from build123d import *

# Parameters (mm, degrees)
F1_DEPTH     = 3
F2_DEPTH     = 8
F3_R         = 8
F4_T4_DEPTH  = 113.9006842239
F4_T9_ANGLE  = 95
F4_T14_ANGLE = 85
F4_T19_DEPTH = 49.1871720396
F4_T24_ANGLE = 95
F4_T29_DEPTH = 20.662188907
F4_T34_ANGLE = 31.4669762933
F4_T39_ANGLE = 62.9339525865
F4_T44_ANGLE = 31.4669762933
F4_T49_DEPTH = 22.2455379196
F4_T54_ANGLE = 85
F4_T59_DEPTH = 49.1871720396
F5_SIZE      = 1
F6_T1_DEPTH  = 123.9388825993
F6_T3_DEPTH  = 59.2253704151
F6_T5_DEPTH  = 42.8508484491
F6_T7_DEPTH  = 59.2253704151
F6_T9_DEPTH  = 43.5593108265
F6_T12_ANGLE = 96.9904356043
F6_T14_ANGLE = 95
F6_T16_ANGLE = 85
F6_T18_ANGLE = 95
F6_T20_ANGLE = 85


# Not quite as in the source:
# - a fillet or chamfer that OpenCascade refuses, or shapes differently, is made with other operations: its cross-section is extruded or revolved along the edge and cut away or added


with BuildPart() as f1:
    # F0 (on Right) → F1 (new body)
    with BuildSketch(Plane.YZ):
        with BuildLine():
            Line((-76.6886542646, 55.3186824411), (-76.6886542646, -19.9678053747))
            Line((-76.6886542646, -19.9678053747), (-38.1131050777, -16.5928821315))
            ThreePointArc((-38.1131050777, -16.5928821315), (-7.4822201157, -3.8748285682), (24.8917797013, -11.0806689666))
            Line((24.8917797013, -11.0806689666), (62.7786034683, -7.76600139))
            Line((62.7786034683, -7.76600139), (62.7786034683, 67.5204864257))
            Line((62.7786034683, 67.5204864257), (-76.6886542646, 55.3186824411))
        make_face()
        with BuildLine():
            Line((-40.0864817191, -11.7464310288), (-71.6886542646, -14.5112628693))
            Line((-71.6886542646, -14.5112628693), (-71.6886542646, 50.737026571))
            Line((-71.6886542646, 50.737026571), (57.7786034683, 62.0639439204))
            Line((57.7786034683, 62.0639439204), (57.7786034683, -3.1843455199))
            Line((57.7786034683, -3.1843455199), (25.9935989152, -5.9651730884))
            ThreePointArc((25.9935989152, -5.9651730884), (-7.9179988294, 1.1061449223), (-40.0864817191, -11.7464310288))
        make_face(mode=Mode.SUBTRACT)
        with BuildLine():
            Line((-71.6886542646, 50.737026571), (-71.6886542646, -14.5112628693))
            Line((-71.6886542646, -14.5112628693), (-40.0864817191, -11.7464310288))
            ThreePointArc((-40.0864817191, -11.7464310288), (-7.9179988294, 1.1061449223), (25.9935989152, -5.9651730884))
            Line((25.9935989152, -5.9651730884), (57.7786034683, -3.1843455199))
            Line((57.7786034683, -3.1843455199), (57.7786034683, 62.0639439204))
            Line((57.7786034683, 62.0639439204), (-71.6886542646, 50.737026571))
        make_face()
    extrude(amount=-F1_DEPTH)

    # F0 (on Right) → F2 (join)
    with BuildSketch(Plane.YZ):
        with BuildLine():
            Line((-71.6886542646, 50.737026571), (-71.6886542646, -14.5112628693))
            Line((-71.6886542646, -14.5112628693), (-40.0864817191, -11.7464310288))
            ThreePointArc((-40.0864817191, -11.7464310288), (-7.9179988294, 1.1061449223), (25.9935989152, -5.9651730884))
            Line((25.9935989152, -5.9651730884), (57.7786034683, -3.1843455199))
            Line((57.7786034683, -3.1843455199), (57.7786034683, 62.0639439204))
            Line((57.7786034683, 62.0639439204), (-71.6886542646, 50.737026571))
        make_face()
    extrude(amount=-F2_DEPTH)

    # F3
    f3_edges = [f1.edges().sort_by_distance(p)[0] for p in [
        (-5.5, 57.778603, 62.063944),
        (-5.5, -71.688654, 50.737027),
        (-5.5, -71.688654, -14.511263),
        (-5.5, -40.086482, -11.746431),
        (-5.5, 25.993599, -5.965173),
        (-5.5, 57.778603, -3.184346),
        (-1.5, -76.688654, 55.318682),
        (-1.5, -76.688654, -19.967805),
        (-1.5, 62.778603, -7.766001),
        (-1.5, 62.778603, 67.520486),
    ]]
    fillet(f3_edges, radius=F3_R)

    # F4: chamfer of 1 x 6 on 1 edges, made by hand


with BuildPart() as f4_tool2:
    # F4_s3 → F4_t4 (new body)
    with BuildSketch(Plane(origin=(0, 54.0311094993, 4.7271095589), x_dir=(1, 0, 0), z_dir=(0, -0.9961946981, -0.0871557427))):
        Polygon((-2, 56.792034776), (-8, 55.792034776), (-8, 56.792034776), align=None)
    extrude(amount=F4_T4_DEPTH)

    split(bisect_by=Plane.YZ.offset(-3), keep=Keep.BOTTOM)


with BuildPart() as f1_1:
    add(f1.part)

    # F4_t1: cut F4_tool2
    add(f4_tool2.part, mode=Mode.SUBTRACT)


with BuildPart() as f4_tool7:
    # F4_s8 → F4_t9 (revolve)
    with BuildSketch(Plane.XY.offset(53.3334759118)):
        Polygon((-2, 57.7786034683), (-8, 56.7786034683), (-8, 57.7786034683), align=None)
    revolve(axis=Axis((-8, 49.7786034683, 53.3334759118), (1, 0, 0)), revolution_arc=F4_T9_ANGLE)

    split(bisect_by=Plane.YZ.offset(-3), keep=Keep.BOTTOM)


with BuildPart() as f1_2:
    add(f1_1.part)

    # F4_t6: cut F4_tool7
    add(f4_tool7.part, mode=Mode.SUBTRACT)


with BuildPart() as f4_tool12:
    # F4_s13 → F4_t14 (revolve)
    with BuildSketch(Plane.XY.offset(43.4063771788)):
        Polygon((-2, -71.6886542646), (-8, -70.6886542646), (-8, -71.6886542646), align=None)
    revolve(axis=Axis((-8, -63.6886542646, 43.4063771788), (-1, 0, 0)), revolution_arc=F4_T14_ANGLE)

    split(bisect_by=Plane.YZ.offset(-3), keep=Keep.BOTTOM)


with BuildPart() as f1_3:
    add(f1_2.part)

    # F4_t11: cut F4_tool12
    add(f4_tool12.part, mode=Mode.SUBTRACT)


with BuildPart() as f4_tool17:
    # F4_s18 → F4_t19 (new body)
    with BuildSketch(Plane.XY.offset(43.4063771788)):
        Polygon((-2, -71.6886542646), (-8, -70.6886542646), (-8, -71.6886542646), align=None)
    extrude(amount=-F4_T19_DEPTH)

    split(bisect_by=Plane.YZ.offset(-3), keep=Keep.BOTTOM)


with BuildPart() as f1_4:
    add(f1_3.part)

    # F4_t16: cut F4_tool17
    add(f4_tool17.part, mode=Mode.SUBTRACT)


with BuildPart() as f4_tool22:
    # F4_s23 → F4_t24 (revolve)
    with BuildSketch(Plane.XY.offset(-5.7807948608)):
        Polygon((-2, -71.6886542646), (-8, -70.6886542646), (-8, -71.6886542646), align=None)
    revolve(axis=Axis((-8, -63.6886542646, -5.7807948608), (1, 0, 0)), revolution_arc=F4_T24_ANGLE)

    split(bisect_by=Plane.YZ.offset(-3), keep=Keep.BOTTOM)


with BuildPart() as f1_5:
    add(f1_4.part)

    # F4_t21: cut F4_tool22
    add(f4_tool22.part, mode=Mode.SUBTRACT)


with BuildPart() as f4_tool27:
    # F4_s28 → F4_t29 (new body)
    with BuildSketch(Plane(origin=(0, -63.7067796281, -5.5736210072), x_dir=(1, 0, 0), z_dir=(0, 0.9961946981, 0.0871557427))):
        Polygon((-2, 8.207965224), (-8, 7.207965224), (-8, 8.207965224), align=None)
    extrude(amount=F4_T29_DEPTH)

    split(bisect_by=Plane.YZ.offset(-3), keep=Keep.BOTTOM)


with BuildPart() as f1_6:
    add(f1_5.part)

    # F4_t26: cut F4_tool27
    add(f4_tool27.part, mode=Mode.SUBTRACT)


with BuildPart() as f4_tool32:
    # F4_s33 → F4_t34 (revolve)
    with BuildSketch(Plane(origin=(0, -43.123216588, -3.7727925862), x_dir=(1, 0, 0), z_dir=(0, -0.9961946981, -0.0871557427))):
        Polygon((-2, -8.207965224), (-8, -7.207965224), (-8, -8.207965224), align=None)
    revolve(axis=Axis((-8, -43.1050912244, -3.9799664398), (1, 0, 0)), revolution_arc=F4_T34_ANGLE)

    split(bisect_by=Plane.YZ.offset(-3), keep=Keep.BOTTOM)


with BuildPart() as f1_7:
    add(f1_6.part)

    # F4_t31: cut F4_tool32
    add(f4_tool32.part, mode=Mode.SUBTRACT)


with BuildPart() as f4_tool37:
    # F4_s38 → F4_t39 (revolve)
    with BuildSketch(Plane(origin=(0, -29.7800133865, -22.0094994379), x_dir=(1, 0, 0), z_dir=(0, -0.8041995665, -0.5943593671))):
        Polygon((-2, 14.4192274514), (-8, 15.4192274514), (-8, 14.4192274514), align=None)
    revolve(axis=Axis((-8, -2.6886542646, -58.6655369632), (-1, 0, 0)), revolution_arc=F4_T39_ANGLE)

    split(bisect_by=Plane.YZ.offset(-3), keep=Keep.BOTTOM)


with BuildPart() as f1_8:
    add(f1_7.part)

    # F4_t36: cut F4_tool37
    add(f4_tool37.part, mode=Mode.SUBTRACT)


with BuildPart() as f4_tool42:
    # F4_s43 → F4_t44 (revolve)
    with BuildSketch(Plane(origin=(0, 21.2512251902, -10.5801809941), x_dir=(1, 0, 0), z_dir=(0, -0.895191389, 0.4456819235))):
        Polygon((-2, 6.2848318723), (-8, 7.2848318723), (-8, 6.2848318723), align=None)
    revolve(axis=Axis((-8, 27.6177165365, 2.207477492), (1, 0, 0)), revolution_arc=F4_T44_ANGLE)

    split(bisect_by=Plane.YZ.offset(-3), keep=Keep.BOTTOM)


with BuildPart() as f1_9:
    add(f1_8.part)

    # F4_t41: cut F4_tool42
    add(f4_tool42.part, mode=Mode.SUBTRACT)


with BuildPart() as f4_tool47:
    # F4_s48 → F4_t49 (new body)
    with BuildSketch(Plane(origin=(0, 27.599591173, 2.4146513456), x_dir=(1, 0, 0), z_dir=(0, 0.9961946981, 0.0871557427))):
        Polygon((-2, 8.207965224), (-8, 7.207965224), (-8, 8.207965224), align=None)
    extrude(amount=F4_T49_DEPTH)

    split(bisect_by=Plane.YZ.offset(-3), keep=Keep.BOTTOM)


with BuildPart() as f1_10:
    add(f1_9.part)

    # F4_t46: cut F4_tool47
    add(f4_tool47.part, mode=Mode.SUBTRACT)


with BuildPart() as f4_tool52:
    # F4_s53 → F4_t54 (revolve)
    with BuildSketch(Plane(origin=(0, 49.7604781047, 4.3534777258), x_dir=(1, 0, 0), z_dir=(0, -0.9961946981, -0.0871557427))):
        Polygon((-2, -8.207965224), (-8, -7.207965224), (-8, -8.207965224), align=None)
    revolve(axis=Axis((-8, 49.7786034683, 4.1463038722), (1, 0, 0)), revolution_arc=F4_T54_ANGLE)

    split(bisect_by=Plane.YZ.offset(-3), keep=Keep.BOTTOM)


with BuildPart() as f1_11:
    add(f1_10.part)

    # F4_t51: cut F4_tool52
    add(f4_tool52.part, mode=Mode.SUBTRACT)


with BuildPart() as f4_tool57:
    # F4_s58 → F4_t59 (new body)
    with BuildSketch(Plane.XY.offset(4.1463038722)):
        Polygon((-2, 57.7786034683), (-8, 56.7786034683), (-8, 57.7786034683), align=None)
    extrude(amount=F4_T59_DEPTH)

    split(bisect_by=Plane.YZ.offset(-3), keep=Keep.BOTTOM)


with BuildPart() as f1_12:
    add(f1_11.part)

    # F4_t56: cut F4_tool57
    add(f4_tool57.part, mode=Mode.SUBTRACT)

    # F5
    f5_edges = [f1_12.edges().sort_by_distance(p)[0] for p in [
        (-8, -7.565116, 55.343289),
        (-8, -68.849596, 48.135509),
        (-8, 54.507735, 58.494417),
        (-8, 54.939545, -0.582828),
        (-8, 39.30825, -3.796472),
        (-8, 26.31403, -4.670051),
        (-8, -8.005155, 2.10234),
        (-8, -40.626941, -10.526627),
        (-8, -52.786783, -11.853744),
        (-8, -68.417786, -10.941736),
        (-8, -70.688654, 18.812791),
        (-8, 56.778603, 28.73989),
    ]]
    chamfer(f5_edges, length=F5_SIZE)

    # F6: chamfer of 5 on 2 edges, made by hand

    # F6_s2 → F6_t1 (cut)
    with BuildSketch(Plane(origin=(0, 59.4668882131, 5.2026785738), x_dir=(1, 0, 0), z_dir=(0, -0.9961946981, -0.0871557427))):
        Polygon((-5, 61.792034776), (0, 56.792034776), (0, 61.792034776), align=None)
    extrude(amount=F6_T1_DEPTH, mode=Mode.SUBTRACT)

    # F6_s4 → F6_t3 (cut)
    with BuildSketch(Plane.XY.offset(-11.2373373661)):
        Polygon((-5, -76.6886542646), (0, -71.6886542646), (0, -76.6886542646), align=None)
    extrude(amount=F6_T3_DEPTH, mode=Mode.SUBTRACT)

    # F6_s6 → F6_t5 (cut)
    with BuildSketch(Plane(origin=(0, -69.1425583419, -6.0491900221), x_dir=(1, 0, 0), z_dir=(0, 0.9961946981, 0.0871557427))):
        Polygon((-5, 13.207965224), (0, 8.207965224), (0, 13.207965224), align=None)
    extrude(amount=F6_T5_DEPTH, mode=Mode.SUBTRACT)

    # F6_s8 → F6_t7 (cut)
    with BuildSketch(Plane.XY.offset(-0.4353519979)):
        Polygon((-5, 62.7786034683), (0, 57.7786034683), (0, 62.7786034683), align=None)
    extrude(amount=F6_T7_DEPTH, mode=Mode.SUBTRACT)

    # F6_s10 → F6_t9 (cut)
    with BuildSketch(Plane(origin=(0, 10.9311448931, 0.9563512575), x_dir=(1, 0, 0), z_dir=(0, 0.9961946981, 0.0871557427))):
        Polygon((-5, 13.207965224), (0, 8.207965224), (0, 13.207965224), align=None)
    extrude(amount=F6_T9_DEPTH, mode=Mode.SUBTRACT)

    # F6_s11 → F6_t12 (revolve, cut)
    with BuildSketch(Plane(origin=(0, -29.0039957446, -39.1898093404), x_dir=(1, 0, 0), z_dir=(0, -0.5948898787, -0.8038072109))):
        Polygon((-5, 22.2616255192), (0, 27.2616255192), (0, 22.2616255192), align=None)
    revolve(axis=Axis((0, -2.6886542646, -58.6655369632), (-1, 0, 0)), revolution_arc=F6_T12_ANGLE, mode=Mode.SUBTRACT)

    # F6_s13 → F6_t14 (revolve, cut)
    with BuildSketch(Plane(origin=(0, 59.4668882131, 5.2026785738), x_dir=(1, 0, 0), z_dir=(0, -0.9961946981, -0.0871557427))):
        Polygon((-5, 61.792034776), (0, 56.792034776), (0, 61.792034776), align=None)
    revolve(axis=Axis((0, 54.7786034683, 58.7900184172), (-1, 0, 0)), revolution_arc=F6_T14_ANGLE, mode=Mode.SUBTRACT)

    # F6_s15 → F6_t16 (revolve, cut)
    with BuildSketch(Plane.XY.offset(47.9880330489)):
        Polygon((-5, -76.6886542646), (0, -71.6886542646), (0, -76.6886542646), align=None)
    revolve(axis=Axis((0, -68.6886542646, 47.9880330489), (-1, 0, 0)), revolution_arc=F6_T16_ANGLE, mode=Mode.SUBTRACT)

    # F6_s17 → F6_t18 (revolve, cut)
    with BuildSketch(Plane.XY.offset(-11.2373373661)):
        Polygon((-5, -76.6886542646), (0, -71.6886542646), (0, -76.6886542646), align=None)
    revolve(axis=Axis((0, -68.6886542646, -11.2373373661), (1, 0, 0)), revolution_arc=F6_T18_ANGLE, mode=Mode.SUBTRACT)

    # F6_s19 → F6_t20 (revolve, cut)
    with BuildSketch(Plane.XY.offset(-0.4353519979)):
        Polygon((-5, 62.7786034683), (0, 57.7786034683), (0, 62.7786034683), align=None)
    revolve(axis=Axis((0, 54.7786034683, -0.4353519979), (-1, 0, 0)), revolution_arc=F6_T20_ANGLE, mode=Mode.SUBTRACT)


solid = f1_12.part
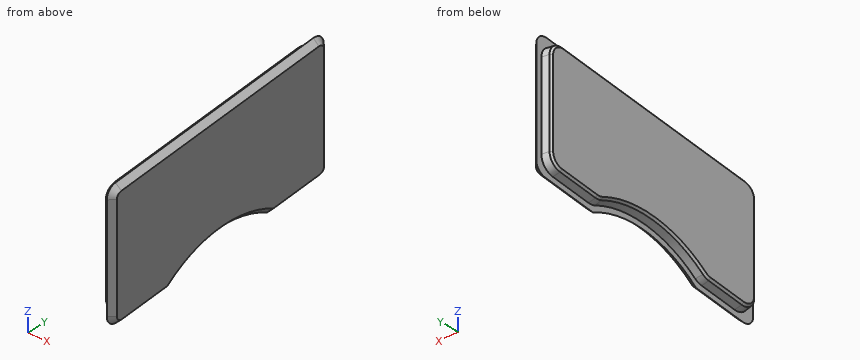
The listing builds one solid part. Answer for the finished solid, in the listing's coordinates (mm). Round coordinates to 2 decimals unless told otherwise and drop trailing zeros. Write each loop counter-clockwise with the first axis right and the second up, starting at its lowest first coordinate (ties: lowest second). Pieces come first, ordered by that corner, then holes. Notation, with made-up numbers: M -30.75,3.25 L -11.75,3.25 A22 ccw -11.75,18.25 Z; hole C -2,20 d8. An arc over 180 degrees is marked long. Write each question's results on one line, items separated by ' | '. Start each with the question number.
(1) The part is cut by section A-A, the plane z = 37.5. Write down the section's boundary in (x, y), and give its area (3 significant figures).
(2) The part is cut by section C-C, the plane y = -44.5. Write down the section's boundary in (x, z), and give its area (3 significant figures).
(3) Find the intervals of material crossed by line 1 (Z direction, x = -5.5, y = -26.5); line 2 (Y direction, x = -5.5, z = 18.5); line 3 (Z direction, x = -2, y = 11.5), in increasing order.
(4) Each of these flat-tipped pins is pushed along its axis until it touches: P1, Ø3, axis at x = -5.5, y = -48.5, coming from the +Z side; P2, Ø2, axis at x = -1, y = -13.5, coming from the -Z side. Where does it stop, or does it pass through?
Worked answers:
1) outline: M -8,-69.69 L -7.01,-70.85 L -3,-71.52 L -3,-74.69 L 0,-71.69 L 0,57.78 L -3,60.78 L -3,57.61 L -7.01,56.94 L -8,55.78 Z | area: 1,040 mm²
2) outline: M -8,-10.12 L -7.01,-11.29 L -3,-11.97 L -3,-15.14 L 0,-12.13 L 0,53.12 L -3,56.13 L -3,52.95 L -7.01,52.28 L -8,51.11 Z | area: 524 mm²
3) line 1: z = -2.96 to 54.1 | line 2: y = -71.11 to 57.2 | line 3: z = -2.43 to 60.02
4) P1: stops at z = 52.46 | P2: stops at z = -1.7
